For this review, use the dimensioned drawing (mm, ordinates from the lowest corner) and the shaded views. A direction names the side the tool comes from. Coordinates: 2 decimals unless noted, no trailing zeros. Write each loop counter-clockwise with the first axis right and the second up, starting at its lowest first coordinate (ties: lowest second). Pieces come first, ordered by that corner, then holes. Notation, with made-up numbers: M -27,-29 L 30,-29 A17 cw 30,-13 Z; hole C 67,54.25 d4. An arc over 180 degrees is marked long. One line per question, with ' | ' between items.
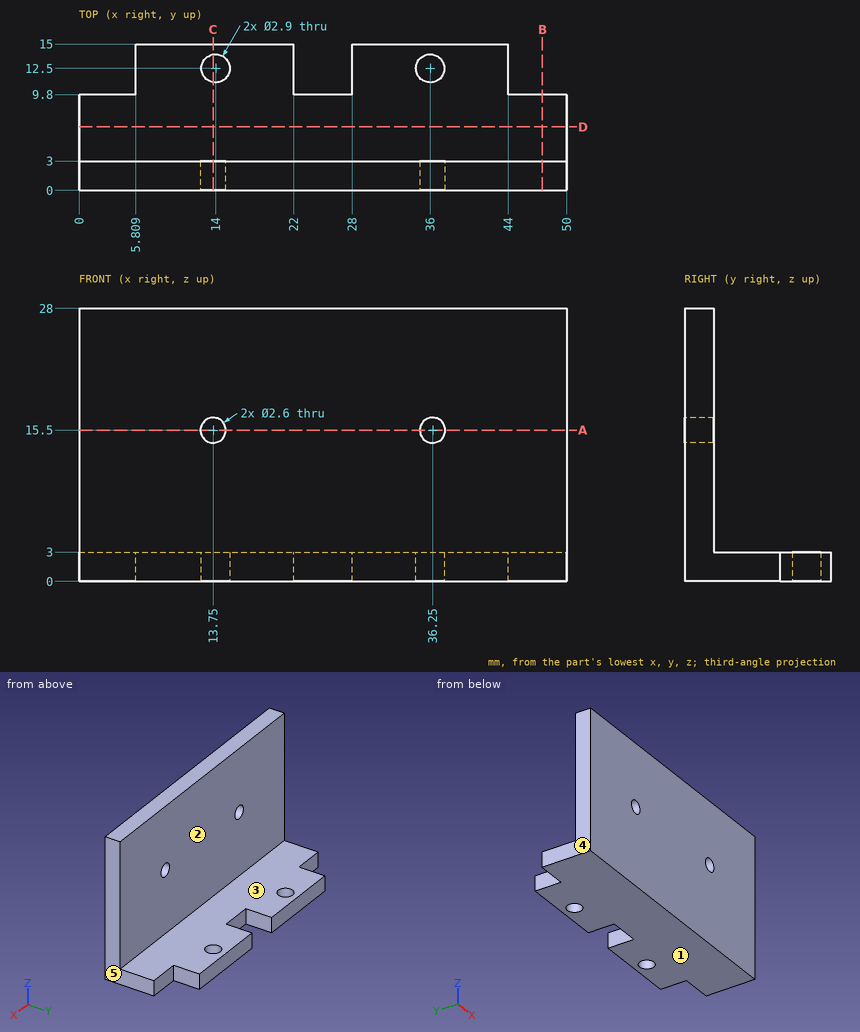
1) The part is to be moulded in two halves that separate along X. For the marked faces 3, 4 and 5, say which applies: +X half, -X half, draft (parallel to the pull), parting line (faces both ways), or undercut.
Responses:
face 3: draft | face 4: -X half | face 5: +X half
2) To check wall thickness, follow line 1 along Y through (x, z) = (14, 2.4); line 2 along Z through (x, y) = (36.25, 1.85); line 3 along Y through (x, z) = (26, 9). State the ranges of each line that lie inside material, in increasing order. Write a range as [from, to].
Responses:
line 1: [0, 11.05], [13.95, 15] | line 2: [0, 14.2], [16.8, 28] | line 3: [0, 3]
3) We need section D-D on y = 6.5. State the section outline as (x, z) points, then the cut area to 3 significant figures.
Responses:
outline: M 0,0 L 50,0 L 50,3 L 0,3 Z | area: 150 mm^2
4) We need section A-A on z = 15.5. State the section outline as (x, y) points, then the cut area to 3 significant figures.
Responses:
outline: M 0,0 L 12.45,0 L 12.45,3 L 0,3 Z; M 15.05,0 L 34.95,0 L 34.95,3 L 15.05,3 Z; M 37.55,0 L 50,0 L 50,3 L 37.55,3 Z | area: 134 mm^2
5) Machinability: for the marked faces 1 and 2, which of the approach directions +Z, -Z, +X, -X, +Y, -Y give a long, thin tool a straight path to every point of the face, cutting with its end or side? Answer none if there is none.
Responses:
face 1: -Z, +X, -X, +Y, -Y | face 2: +Z, +X, -X, +Y
6) We need section B-B on x = 47.5. State the section outline as (y, z) points.
Responses:
outline: M 0,0 L 9.8,0 L 9.8,3 L 3,3 L 3,28 L 0,28 Z
7) Insertion check: pin 1 Ø1.5 at (x, z) = (44, 24.5) entering from +Y; pin 2 Ø3.5 at (y, z) = (13.5, 1.5) entering from +X; pin 3 Ø0.9 at (x, z) = (48.5, 2) entering from +Y. Each pin has a flat end and moves straight along its axis. Give the tip position at first contact, or say it passes through.
Responses:
pin 1: y = 3 | pin 2: x = 44 | pin 3: y = 9.8
8) We need section C-C on x = 13.75. State the section outline as (y, z) points.
Responses:
outline: M 0,0 L 11.07,0 L 11.07,3 L 3,3 L 3,14.2 L 0,14.2 Z; M 0,16.8 L 3,16.8 L 3,28 L 0,28 Z; M 13.93,0 L 15,0 L 15,3 L 13.93,3 Z
